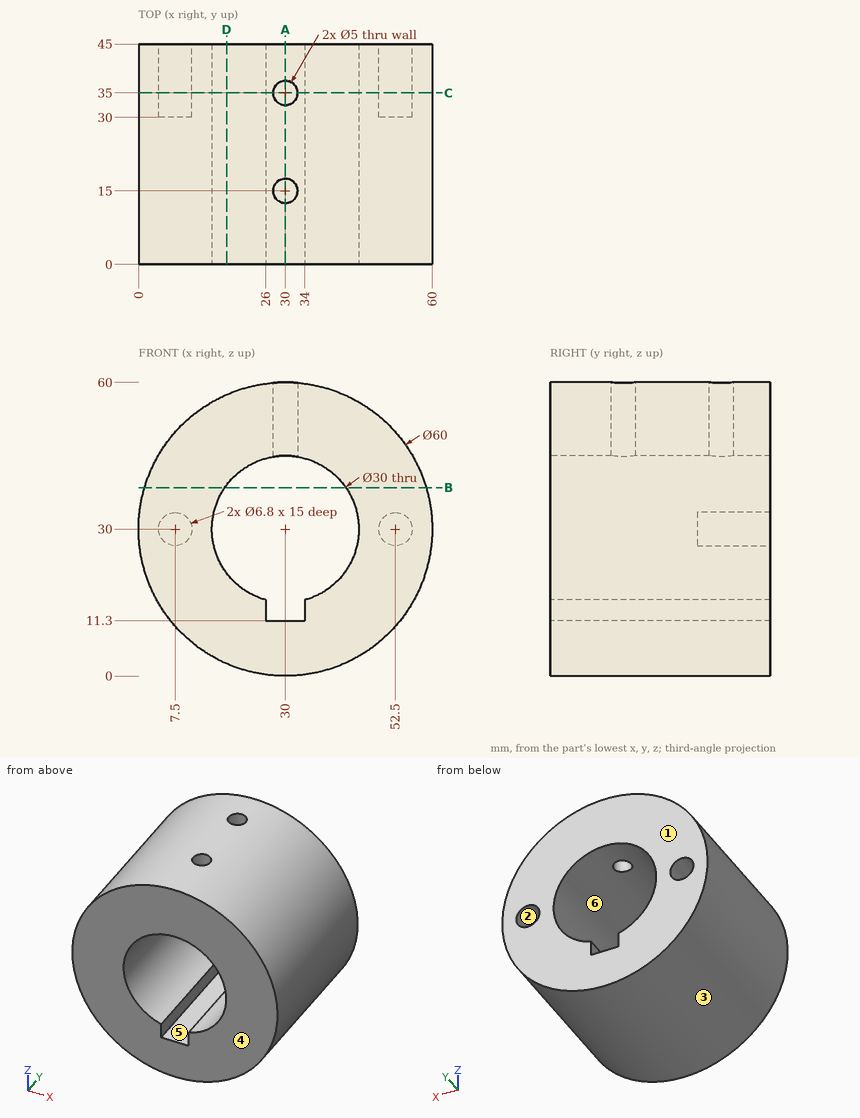
Check sheet for the drawn part. Datum: minimum x, y, z corner. Units: mm. A direction names the side the tool comes from. Coordinates: 2 decimals unless noted, no trailing zeros. Order: outer loops, then holes, each group sorted by start corner. A loop starts at its lowest first (then second) coordinate and runs counter-clockwise, first axis right, second up. Notation, with made-up numbers: M 13.5,-5 L 19.5,-5 A37 ccw 19.5,33 Z; hole C -32.75,61 d4. An arc over 180 degrees is marked long. One line per question, with ' | ' between items. Start each with the question number.
Item 1: Cross-section at B-B on z = 38.5. Enter the section's corners in (x, y), then the cut area to 3 significant figures.
Item 2: Material ranges on L1, parallel to X at y = 36.5, z = 30; L2, parallel to Z at x = 7, y = 35; L3, parallel to X at y = 16.5, z = 50, recorded low to high. Write a range as [from, to].
Item 3: Cross-section at D-D on x = 18. Enter the section's corners in (y, z), then the cut area to 3 significant figures.
Item 4: Cross-section at C-C on y = 35. Enter the section's corners in (x, z).
Item 5: Gauge pin test, flat ends, axial feed: pin 1 (6 mm diameter, centred on y = 21, z = 17, fed in from +X); pin 2 (12 mm diameter, centred on x = 49, y = 24, fed in from +Z); pin 3 (3 mm diameter, centred on x = 21, y = 30, fed in from +Z). Record the tip position at first contact, or that the pin passes through.
Item 6: Set-up check for the marked faces 1 and 2: record each of +Z, -Z, +X, -X, +Y, -Y from which the full face is reachable in a straight line by a thin tool's end or side.
Item 7: Cross-section at A-A on x = 30. Enter the section's corners in (y, z).
Item 8: Draft check along X on the marked faces 3, 4, 5 and 6. Enter one of: pulls with the +X half, pulls with the -X half, needs draft (parallel to the pull), parting line crosses it, or undercut.
Findings:
1) outline: M 1.23,0 L 17.64,0 L 17.64,45 L 1.23,45 Z; M 42.36,0 L 58.77,0 L 58.77,45 L 42.36,45 Z | area: 1,480 mm²
2) L1: x = [0, 4.1], [10.9, 15], [45, 49.1], [55.9, 60] | L2: z = [10.74, 26.64], [33.36, 49.26] | L3: x = [7.64, 28], [32, 52.36]
3) outline: M 0,2.5 L 45,2.5 L 45,21 L 0,21 Z; M 0,39 L 45,39 L 45,57.5 L 0,57.5 Z | area: 1,660 mm²
4) outline: M 26,11.3 L 26,15.54 A15 cw 27.5,44.79 L 27.5,59.9 A30 ccw long 32.5,59.9 L 32.5,44.79 A15 cw 34,15.54 L 34,11.3 Z; hole C 7.5,30 d6.8; hole C 52.5,30 d6.8
5) pin 1: stops at x = 58.28 | pin 2: stops at z = 57.04 | pin 3: stops at z = 59.05
6) face 1: +Z, -Z, +X, -X, +Y | face 2: +Y
7) outline: M 0,0 L 45,0 L 45,11.3 L 0,11.3 Z; M 0,45 L 12.5,45 L 12.5,60 L 0,60 Z; M 17.5,45 L 32.5,45 L 32.5,60 L 17.5,60 Z; M 37.5,45 L 45,45 L 45,60 L 37.5,60 Z
8) face 3: parting line crosses it | face 4: needs draft | face 5: undercut | face 6: undercut
